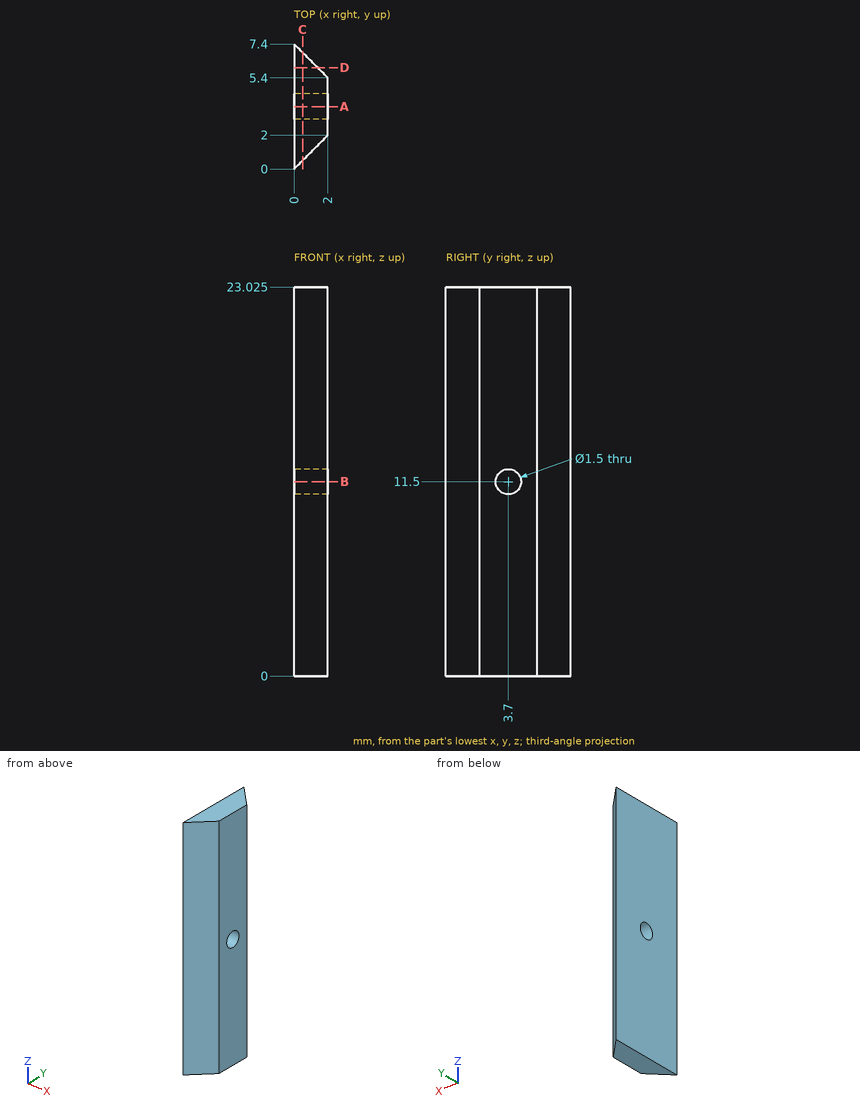
Verification items for this drawing (mm, ordinates from the low corner). Give positions to 0.01 mm unless a question says otherwise; leave off trailing zeros. Write each loop counter-clockwise with the first axis right and the second up, starting at its lowest first coordinate (ties: lowest second). Pieces come first, ordered by that corner, then holes. Notation, with made-up numbers: (84.5, 57) - (105.5, 57) arc R13 ccw to (105.5, 67) - close; hole circle Ø11 at (24.5, -31). An arc over 180 degrees is marked (long way). Answer as a JSON object with one key per item and string values. Group by question number.
1) Sectioned sample at D-D (y = 6). Record the cut outline in (x, z) (3 decimals).
2) Sectioned sample at C-C (x = 0.5). Record the cut outline in (y, z) (3 decimals), then the cut area to 3 significant figures.
3) Sectioned sample at A-A (y = 3.7). Record the cut outline in (x, z) (3 decimals).
4) Sectioned sample at B-B (z = 11.5). Record the cut outline in (x, y), then the cut area to 3 significant figures.
5) Thickness scan on probe 1 along Z at (x, y) = (0.4, 3.7) (3 decimals); probe 2 along Y at (x, z) = (1.3, 11.25); probe 3 along Y at (x, z) = (0.75, 11.5). Record the ranges inside material, lowest first. Write a range as from..to.
Geometry results:
{
 "1": {"outline": "(0, 0) - (1.4, 0) - (1.4, 23.025) - (0, 23.025) - close"},
 "2": {"outline": "(0.5, 0) - (6.9, 0) - (6.9, 23.025) - (0.5, 23.025) - close; hole circle Ø1.5 at (3.7, 11.5)", "area": "146 mm^2"},
 "3": {"outline": "(0, 0) - (2, 0) - (2, 10.75) - (0, 10.75) - close; (0, 12.25) - (2, 12.25) - (2, 23.025) - (0, 23.025) - close"},
 "4": {"outline": "(0, 0) - (2, 2) - (2, 2.95) - (0, 2.95) - close; (0, 4.45) - (2, 4.45) - (2, 5.4) - (0, 7.4) - close", "area": "7.80 mm^2"},
 "5": {"probe 1": "z = 0..10.75, 12.25..23.025", "probe 2": "y = 1.3..2.99, 4.41..6.1", "probe 3": "y = 0.75..2.95, 4.45..6.65"}
}
